from build123d import *

# Parameters (mm, degrees)
BOSS_EXTRUDE1_DEPTH      = 62
CUT_EXTRUDE1_DEPTH       = 12
CUT_EXTRUDE1_DEPTH_BACK  = 12
BOSS_EXTRUDE2_DEPTH      = 1
BOSS_EXTRUDE2_DEPTH_BACK = 1.5
CUT_EXTRUDE3_DEPTH       = 10
CHAMFER2_SIZE            = 2
CHAMFER3_SIZE            = 2
CHAMFER4_SIZE            = 4
CHAMFER4_SIZE2           = 6.92820323
SKETCH7_R                = 4
CUT_EXTRUDE4_DEPTH       = 70
CUT_EXTRUDE5_REACH       = 87.071
SKETCH8_R                = 1.5


with BuildPart() as part:
    # Sketch1 → Boss-Extrude1 (new body)
    with BuildSketch(Plane(origin=(0, 0, 0), x_dir=(0, 0, -1), z_dir=(1, 0, 0))):
        with BuildLine():
            Line((47, -12), (0, -12))
            ThreePointArc((0, -12), (-7.348469228, 9.486832981), (11.618950039, -3))
            Line((11.618950039, -3), (47, -3))
            Line((47, -3), (47, -12))
        make_face()
    extrude(amount=-BOSS_EXTRUDE1_DEPTH)

    # Sketch2 → Cut-Extrude1 (cut, two sides: drawn at the far end of the back side and taken through both)
    with BuildSketch(Plane(origin=(0, 0, 0), x_dir=(1, 0, 0), z_dir=(0, 1, 0)).offset(-CUT_EXTRUDE1_DEPTH_BACK)):
        Polygon((-58, -12), (-58, 43), (-36, 43), (-36, 41), (-26, 41), (-26, 43), (-4, 43), (-4, -12), align=None)
    extrude(amount=CUT_EXTRUDE1_DEPTH + CUT_EXTRUDE1_DEPTH_BACK, mode=Mode.SUBTRACT)

    # Sketch3 → Boss-Extrude2 (add, two sides: drawn at the far end of the back side and taken through both)
    with BuildSketch(Plane(origin=(0, -3, 0), x_dir=(1, 0, 0), z_dir=(0, 1, 0)).offset(-BOSS_EXTRUDE2_DEPTH_BACK)):
        with BuildLine():
            Line((-35.5, 57), (-35.5, 47))
            Line((-35.5, 47), (-26.5, 47))
            Line((-26.5, 47), (-26.5, 57))
            Line((-26.5, 57), (-28.25, 57))
            ThreePointArc((-28.25, 57), (-31, 54.25), (-33.75, 57))
            Line((-33.75, 57), (-35.5, 57))
        make_face()
    extrude(amount=BOSS_EXTRUDE2_DEPTH + BOSS_EXTRUDE2_DEPTH_BACK)

    # Sketch5 → Cut-Extrude3 (cut)
    with BuildSketch(Plane(origin=(0, -3, 0), x_dir=(1, 0, 0), z_dir=(0, 1, 0))):
        with BuildLine():
            Line((-32.35, 43), (-29.65, 43))
            ThreePointArc((-29.65, 43), (-28.65, 44), (-29.65, 45))
            Line((-29.65, 45), (-29.65, 47))
            Line((-29.65, 47), (-32.35, 47))
            Line((-32.35, 47), (-32.35, 45))
            ThreePointArc((-32.35, 45), (-33.35, 44), (-32.35, 43))
        make_face()
    extrude(amount=-CUT_EXTRUDE3_DEPTH, mode=Mode.SUBTRACT)

    # Chamfer2
    chamfer2_edges = [part.edges().sort_by_distance(p)[0] for p in [
        (-26, -7.5, -41),
    ]]
    chamfer(chamfer2_edges, length=CHAMFER2_SIZE - 0.0001)  # a hair under: the kernel refuses the full size

    # Chamfer3
    chamfer3_edges = [part.edges().sort_by_distance(p)[0] for p in [
        (-36, -7.5, -41),
    ]]
    chamfer(chamfer3_edges, length=CHAMFER3_SIZE - 0.0001)  # a hair under: the kernel refuses the full size

    # Chamfer4
    chamfer4_edges = [part.edges().sort_by_distance(p)[0] for p in [
        (-33.925, -4.5, -47),
        (-28.075, -4.5, -47),
    ]]
    chamfer4_side = [part.faces().sort_by_distance(p)[0] for p in [
        (-31, -4.5, -51.417170305),
    ]]
    chamfer(chamfer4_edges, length=CHAMFER4_SIZE, length2=CHAMFER4_SIZE2, reference=chamfer4_side[0])

    # Sketch7 → Cut-Extrude4 (cut)
    with BuildSketch(Plane(origin=(0, 0, 0), x_dir=(0, 0, -1), z_dir=(1, 0, 0))):
        Circle(SKETCH7_R)
    extrude(amount=-CUT_EXTRUDE4_DEPTH, mode=Mode.SUBTRACT)

    # Sketch8 → Cut-Extrude5 (cut, up to next)
    with BuildSketch(Plane.ZY.offset(62), mode=Mode.PRIVATE) as cut_extrude5_sk1:
        with Locations((0, 7)):
            Circle(SKETCH8_R)
    cut_extrude5_tool1 = extrude(cut_extrude5_sk1.sketch, amount=-CUT_EXTRUDE5_REACH, mode=Mode.PRIVATE) & part.part
    # Sketch8 → Cut-Extrude5 (cut, up to next)
    with BuildSketch(Plane.ZY.offset(62), mode=Mode.PRIVATE) as cut_extrude5_sk2:
        with Locations((7, 0)):
            Circle(SKETCH8_R)
    cut_extrude5_tool2 = extrude(cut_extrude5_sk2.sketch, amount=-CUT_EXTRUDE5_REACH, mode=Mode.PRIVATE) & part.part
    # Sketch8 → Cut-Extrude5 (cut, up to next)
    with BuildSketch(Plane.ZY.offset(62), mode=Mode.PRIVATE) as cut_extrude5_sk3:
        with Locations((0, -7)):
            Circle(SKETCH8_R)
    cut_extrude5_tool3 = extrude(cut_extrude5_sk3.sketch, amount=-CUT_EXTRUDE5_REACH, mode=Mode.PRIVATE) & part.part
    # Sketch8 → Cut-Extrude5 (cut, up to next)
    with BuildSketch(Plane.ZY.offset(62), mode=Mode.PRIVATE) as cut_extrude5_sk4:
        with Locations((-7, 0)):
            Circle(SKETCH8_R)
    cut_extrude5_tool4 = extrude(cut_extrude5_sk4.sketch, amount=-CUT_EXTRUDE5_REACH, mode=Mode.PRIVATE) & part.part
    add(cut_extrude5_tool1.solids().sort_by_distance((-62, 7, 0))[0], mode=Mode.SUBTRACT)
    add(cut_extrude5_tool2.solids().sort_by_distance((-62, 0, 7))[0], mode=Mode.SUBTRACT)
    add(cut_extrude5_tool3.solids().sort_by_distance((-62, -7, 0))[0], mode=Mode.SUBTRACT)
    add(cut_extrude5_tool4.solids().sort_by_distance((-62, 0, -7))[0], mode=Mode.SUBTRACT)


solid = part.part
The model under review builds one solid part; all positions refer to its coordinate system, in mm. A direction names the side the tool comes from. Give positions to 0.01 mm unless a question says otherwise; leave off trailing zeros. Write each loop counter-clockwise with the first axis right and the second up, starting at its lowest first coordinate (ties: lowest second). Pieces come first, ordered by that corner, then holes.
1. Draft analysis for pull direction Z (two halves, no side actions). For faces 6 (the cylindrical face through (-60.03, 0.07, 5.5)), 7 (the flat face through (-30.9, -12, -42.8)), 8 (the flat face through (-33.947, -8.013, -48.972)), state which applies: +Z half, -Z half, draft (parallel to the pull), parting line (faces both ways), or undercut.
2. Add section D-D, the plane z = 7. Write out the cut boundary in (x, y), plus the area to 3 significant figures.
3. Add section A-A, the plane z = -34. Write out the cut boundary in (x, y), plus the area to 3 significant figures.
4. Tool access review of faces 1 (the flat face through (-31, -3, -47)), 2 (the flat face through (-35.5, -5, -50)), 3 (the flat face through (-29.65, -7, -47)), 4 (the cylindrical face through (-33.35, -7.44, -44.02)), 5 (the cylindrical face through (-60.028, 5.536, -0.325)): name each direction out of +Z, -Z, +X, -X, +Y, -Y from which nothing blocks a thin tool from reaching the whole face with its end or side.
5. Add section C-C, the plane y = 0. Write out the cut boundary in (x, z).
6. For P1, Ø2.5, axis at y = -7, z = 0, coming from the -X side; P2, Ø12, axis at x = -56, y = -0.5, coming from the -Z side; P3, Ø3, axis at x = -53.5, y = -1, coming from the -Z side; P4, Ø8, axis at x = -31.5, y = -8, coming from the +Z side, all flat-tipped, find the tip position at first contact; note any pin that passes through.
7. Wall thickness on L1, parallel to Y at x = -60.25, z = 0; L2, parallel to X at y = -7.75, z = -28; L3, parallel to X at y = -10, z = -44: over which ranges is each line inside the solid? List them lowest first.
8. Add section B-B, the plane x = -31. Write out the cut boundary in (y, z).
Worked answers:
1. face 6: undercut
1. face 7: draft
1. face 8: -Z half
2. outline: (-62, -9.75) - (-58, -9.75) - (-58, -1.5) - (-62, -1.5) - close; (-62, 1.5) - (-58, 1.5) - (-58, 9.75) - (-62, 9.75) - close; (-4, -9.75) - (0, -9.75) - (0, 9.75) - (-4, 9.75) - close
2. area: 144 mm2
3. outline: (-62, -12) - (-58, -12) - (-58, -3) - (-62, -3) - close; (-4, -12) - (0, -12) - (0, -3) - (-4, -3) - close
3. area: 72.0 mm2
4. face 1: +Y
4. face 2: -Z, -X, +Y, -Y
4. face 3: -Y
4. face 4: +Y, -Y
4. face 5: -X
5. outline: (-62, -12) - (-58, -12) - (-58, -8.5) - (-62, -8.5) - close; (-62, -5.5) - (-58, -5.5) - (-58, -4) - (-62, -4) - close; (-62, 4) - (-58, 4) - (-58, 5.5) - (-62, 5.5) - close; (-62, 8.5) - (-58, 8.5) - (-58, 12) - (-62, 12) - close; (-4, -12) - (0, -12) - (0, -4) - (-4, -4) - close; (-4, 4) - (0, 4) - (0, 12) - (-4, 12) - close
6. P1: stops at x = -4
6. P2: stops at z = -47
6. P3: passes through
6. P4: stops at z = -41
7. L1: y = -12 to -8.5, -5.5 to -4, 4 to 5.5, 8.5 to 12
7. L2: x = -62 to -58, -4 to 0
7. L3: x = -62 to -33.35, -28.65 to 0
8. outline: (-12, -43) - (-3, -43) - (-3, -41) - (-12, -41) - close; (-4.5, -54.25) - (-2, -54.25) - (-2, -47) - (-4.5, -47) - close
